Autodesk Inventor part; units mm, degrees
ref_plane "YZ Plane" through (0, 0, 0) normal (1, 0, 0) x (0, 1, 0)
ref_plane "XZ Plane" through (0, 0, 0) normal (0, 1, 0) x (-1, 0, 0)
ref_plane "XY Plane" through (0, 0, 0) normal (0, 0, 1) x (1, 0, 0)
sketch "Sketch1" plane through (11.7508, -1.15, -2.5) normal (0, 0, -1) x (-1, 0, 0)
  line L0 (0.2594, -0.35) -> (11.8421, -0.35)
  line L1 (11.8421, 9.05) -> (10.9395, 9.05)
  line L2 (1.162, 9.05) -> (0.2594, 9.05)
  line L3 (11.7508, -0.35) -> (0.2594, -0.35)
  line L4 (0.2594, -0.35) -> (0.2594, 9.05)
  line L5 (0.2594, 9.05) -> (11.7508, 9.05)
  line L6 (11.7508, 9.05) -> (11.7508, -0.35)
  point P0 (11.7508, 1.15)
extrude "Extrusion1" add sketch "Sketch1" along normal blind 10
sketch "Sketch2" plane through (0, -1.5, -2.5) normal (0, -1, 0) x (1, 0, 0)
  line L0 (0, 0) -> (0, -10)
  line L1 (11.4914, 0) -> (11.4914, -10)
  line L2 (11.4914, -10) -> (0, -10)
  line L3 (11.4914, 0) -> (0, 0)
  line L4 (0, -10) -> (11.4914, 0)
  circle A0 centre (5.7457, -5) radius 2.5
  point P0 (0, 2.5)
  dimension "d2" = 5
extrude "Extrusion2" add sketch "Sketch2" along normal blind 100 contours A0 L4 | L4 A0
chamfer "Chamfer1" distance 2 distance2 80 1 edges at (3.2457, -1.5, -7.5) measured on face at (10.4095, -1.5, -7.5)
chamfer "Chamfer2" distance 1 angle 45 1 edges at (3.2457, -101.5, -7.5)
sketch "Sketch3" plane through (11.7508, -1.15, -12.5) normal (0, 0, -1) x (-1, 0, 0)
  line L0 (0.2594, 9.05) -> (0.2594, -0.35)
  line L1 (3.0508, 8.8) -> (9.0508, 8.8)
  line L2 (11.7508, 7.55) -> (11.7508, -0.85)
  line L3 (9.0508, 7.55) -> (11.7508, 7.55)
  line L4 (9.0508, 8.8) -> (9.0508, 7.55)
  line L5 (3.0508, 7.55) -> (0.3508, 7.55)
  line L6 (3.0508, 8.8) -> (3.0508, 7.55)
  line L7 (0.3508, 7.55) -> (0.3508, -0.85)
  line L8 (0.3508, 1.15) -> (11.7508, 1.15)
extrude "Extrusion3" add sketch "Sketch3" against normal blind 20.625
properties part number "RJ45 Port Cap_Slim_3DPrint"
Here's how the part is built. I have some questions about the finished solid (model axes, mm). A direction names the side the tool comes from. Round coordinates to 2 decimals unless told otherwise and drop trailing zeros. Write each loop counter-clockwise with the first axis right and the second up, starting at its lowest first coordinate (ties: lowest second). Pieces come first, ordered by that corner, then holes.
Q1. Please list where these lines run through material, in increasing order: probe 1 along Y at (x, z) = (9, 1); probe 2 along Z at (x, y) = (2.25, -0.5); probe 3 along Z at (x, y) = (4, -59.5).
Q2. Will these pins go through, and if not, where does the flat tip stop? P1, Ø4, axis at x = 1.5, y = -83, coming from the +Z side; P2, Ø0.6, axis at y = 7, z = 1, coming from the +X side; P3, Ø5.5, axis at x = 6, z = 5, coming from the -Y side.
Q3. If we section it at C-C on z = -7.5: Write out the boundary of the cut face in (x, y), plus the area to 3 significant figures.
Q4. Which directions (+Z, -Z, +X, -X, +Y, -Y) give clear straight access to the entire face, cutting with the end or side of a thin tool? Please do faces 1 (the flat face through (10, -1.5, -5)), 2 (the flat face through (1, 6.4, 3)), 3 (the flat face through (6, 0, 3)), 4 (the flat face through (11.4, 3, 3)), 5 (the flat face through (10, 6.4, 3)).
Q5. If we section it at B-B on y = -85: Write out the boundary of the cut face in (x, z).
Q6. If we section it at A-A on z = 1.75: Write out the boundary of the cut face in (x, y).
Q7. If we section it at D-D on y = -8: Write out the boundary of the cut face in (x, z) (1 decimal), plus the area to 3 significant figures.
Answer below:
1. probe 1: y = 0 to 6.4
1. probe 2: z = -12.5 to -2.5
1. probe 3: z = -10 to -5
2. P1: stops at z = -6.4
2. P2: stops at x = 8.7
2. P3: stops at y = 0
3. outline: (0, -1.5) - (1.25, -1.5) - (3.25, -81.5) - (3.25, -100.5) - (4.25, -101.5) - (7.25, -101.5) - (8.25, -100.5) - (8.25, -81.5) - (10.25, -1.5) - (11.49, -1.5) - (11.49, 7.9) - (0, 7.9) - close
3. area: 767 mm2
4. face 1: -Y
4. face 2: +Z, -X, +Y
4. face 3: +Z, +X, -X, -Y
4. face 4: +Z, +X, +Y, -Y
4. face 5: +Z, +X, +Y
5. outline: circle Ø5 at (5.75, -7.5)
6. outline: (0, 0) - (11.4, 0) - (11.4, 6.4) - (8.7, 6.4) - (8.7, 7.65) - (2.7, 7.65) - (2.7, 6.4) - (0, 6.4) - close
7. outline: circle Ø8.7 at (5.7, -7.5)
7. area: 59.1 mm2
